Build history of the part. All positions in model axes, mm. A direction names the side the tool comes from. Give positions to 0.01 mm unless a question says otherwise; leave off trailing zeros. Order: outer loops, then holes, each group sorted by start corner. A loop starts at its lowest first (then second) coordinate and runs counter-clockwise, first axis right, second up. Notation, with made-up numbers: (-26.75, -3.5) - (30.25, -3.5) arc R25 ccw to (30.25, 9.5) - close; hole circle Ø3 at (53, 56.25). An arc over 180 degrees is marked (long way). Answer in a Markdown table with one row per item.
```python
from build123d import *

# Parameters (mm, degrees)
SKETCH1_W           = 89
SKETCH1_H           = 83
SKETCH1_R           = 1.3
SKETCH1_W_2         = 15
SKETCH1_H_2         = 30
MAIN_BODY_DEPTH     = 14
SKETCH2_W           = 40
SKETCH2_H           = 83
SCREW_GROOVE_DEPTH  = 6
SKETCH4_W           = 9
SKETCH4_H           = 83
BOSS_EXTRUDE2_DEPTH = 6


with BuildPart() as part:
    # Sketch1 → Main Body (new body)
    with BuildSketch(Plane(origin=(0, 0, 0), x_dir=(1, 0, 0), z_dir=(0, 1, 0))):
        with Locations((0, 41.5)):
            Rectangle(SKETCH1_W, SKETCH1_H)
        with Locations((30, 68.75)):
            Circle(SKETCH1_R, mode=Mode.SUBTRACT)
        with Locations((-30, 68.75)):
            Circle(SKETCH1_R, mode=Mode.SUBTRACT)
        with Locations((-30, 14.25)):
            Circle(SKETCH1_R, mode=Mode.SUBTRACT)
        with Locations((30, 14.25)):
            Circle(SKETCH1_R, mode=Mode.SUBTRACT)
        with Locations((0, 20)):
            Rectangle(SKETCH1_W_2, SKETCH1_H_2, mode=Mode.SUBTRACT)
    extrude(amount=MAIN_BODY_DEPTH)

    # Sketch2 → Screw Groove (cut)
    with BuildSketch(Plane(origin=(0, 14, 0), x_dir=(1, 0, 0), z_dir=(0, 1, 0))):
        with Locations((0, 41.5)):
            Rectangle(SKETCH2_W, SKETCH2_H)
    extrude(amount=-SCREW_GROOVE_DEPTH, mode=Mode.SUBTRACT)

    # Sketch4 → Boss-Extrude2 (add)
    with BuildSketch(Plane(origin=(0, 14, 0), x_dir=(1, 0, 0), z_dir=(0, 1, 0))):
        with Locations((-40, 41.5)):
            Rectangle(SKETCH4_W, SKETCH4_H)
        with Locations((40, 41.5)):
            Rectangle(SKETCH4_W, SKETCH4_H)
    extrude(amount=BOSS_EXTRUDE2_DEPTH)


solid = part.part
```
1. Cut at D-D on z = -68.75. Write the cut outline in (x, y), and give its area (3 significant figures).
Check result:
| item | result |
|---|---|
| outline | (-44.5, 0) - (-31.3, 0) - (-31.3, 14) - (-35.5, 14) - (-35.5, 20) - (-44.5, 20) - close; (-28.7, 0) - (28.7, 0) - (28.7, 14) - (20, 14) - (20, 8) - (-20, 8) - (-20, 14) - (-28.7, 14) - close; (31.3, 0) - (44.5, 0) - (44.5, 20) - (35.5, 20) - (35.5, 14) - (31.3, 14) - close |
| area | 1,040 mm² |
2. Cut at A-A on z = -14.25. Write the cut outline in (x, y).
Check result:
| item | result |
|---|---|
| outline | (-44.5, 0) - (-31.3, 0) - (-31.3, 14) - (-35.5, 14) - (-35.5, 20) - (-44.5, 20) - close; (-28.7, 0) - (-7.5, 0) - (-7.5, 8) - (-20, 8) - (-20, 14) - (-28.7, 14) - close; (7.5, 0) - (28.7, 0) - (28.7, 14) - (20, 14) - (20, 8) - (7.5, 8) - close; (31.3, 0) - (44.5, 0) - (44.5, 20) - (35.5, 20) - (35.5, 14) - (31.3, 14) - close |
3. Probe line 1 (Z direction, x = -30, y = 7.25); line 2 (X direction, y = 4.75, z = -68.75); line 3 (X direction, y = 3.5, z = -14.25). List the from-to ranges inside material, lowest first.
Check result:
| item | result |
|---|---|
| line 1 | z = -83 to -70.05, -67.45 to -15.55, -12.95 to 0 |
| line 2 | x = -44.5 to -31.3, -28.7 to 28.7, 31.3 to 44.5 |
| line 3 | x = -44.5 to -31.3, -28.7 to -7.5, 7.5 to 28.7, 31.3 to 44.5 |
4. Cut at B-B on x = -30. Write the cut outline in (y, z), and give its area (3 significant figures).
Check result:
| item | result |
|---|---|
| outline | (0, -83) - (14, -83) - (14, -70.05) - (0, -70.05) - close; (0, -67.45) - (14, -67.45) - (14, -15.55) - (0, -15.55) - close; (0, -12.95) - (14, -12.95) - (14, 0) - (0, 0) - close |
| area | 1,090 mm² |
5. Which spindle directions (+Z, -Z, +X, -X, +Y, -Y) get a long thin tool onto all of the face, cutting with end or side? Do faces 4 (the face through (0, 4, -35)), 5 (the face through (-44.5, 10, -41)), 6 (the face through (20, 11, -41)). Say none if no direction does.
Check result:
| item | result |
|---|---|
| face 4 | +Y, -Y |
| face 5 | +Z, -Z, -X, +Y, -Y |
| face 6 | +Z, -Z, +Y |
6. Drop flat-ended pins along their axis: P1, Ø12.5, axis at x = 25, z = -22, coming from the +Y side; P2, Ø10, axis at x = -31, z = -42.5, coming from the -Y side. Give the stop position or say it passes through.
Check result:
| item | result |
|---|---|
| P1 | stops at y = 14 |
| P2 | stops at y = 0 |
7. Cut at C-C on y = 6.5. Write the cut outline in (x, z).
Check result:
| item | result |
|---|---|
| outline | (-44.5, -83) - (44.5, -83) - (44.5, 0) - (-44.5, 0) - close; hole circle Ø2.6 at (-30, -68.75); hole circle Ø2.6 at (-30, -14.25); hole (-7.5, -35) - (7.5, -35) - (7.5, -5) - (-7.5, -5) - close; hole circle Ø2.6 at (30, -68.75); hole circle Ø2.6 at (30, -14.25) |
8. Two-plate mould, pull along X, no slides. Class faces 1 (the face through (0, 4, -5)), 2 (the face through (44.5, 10, -41)), 3 (the face through (40, 20, -42)): +X half, -X half, draft (parallel to the pull), parting line (faces both ways), or undercut.
Check result:
| item | result |
|---|---|
| face 1 | undercut |
| face 2 | +X half |
| face 3 | draft |
